Here's how the part is built. I have some questions about the finished solid (model axes, mm). Give positions to 0.01 mm unless a question says otherwise; leave off trailing zeros. Use CSV: the item, a comma, the result in double quotes. Start each with the question number.
(1) For pin 1 Ø2.5 at (x, z) = (50.42, -2.93) entering from -Y, with a flat end and sliding along its axis, tell me the tip position at first contact or that it passes through.
(2) Suppose I cut it at A-A on y = -0.5. Give the number of separate pieces and of enclosed holes in the cut face, plus the area to 3 significant figures.
(3) I need wall thicknesses on L1, parallel to X at y = -0.25, z = 15.5; L2, parallel to X at y = -1.35, z = -19.5; L3, parallel to X at y = -0.1, z = 6.5. Which ranges of each line are inside material? Lowest first, please. Write a range as [from, to].
from build123d import *

# Parameters (mm, degrees)
F0_R     = 1.857944
F0_R_2   = 1.417802
F0_R_3   = 1.435008
F0_R_4   = 1.79954
F0_R_5   = 1.437898
F0_R_6   = 1.231078
F0_R_7   = 1.385876
F0_R_8   = 1.711076
F0_R_9   = 1.741872
F0_R_10  = 1.225641
F0_R_11  = 1.503057
F0_R_12  = 1.860203
F0_R_13  = 1.749094
F0_R_14  = 1.743489
F0_R_15  = 1.494291
F0_R_16  = 1.596373
F0_R_17  = 1.637338
F1_DEPTH = 1.5875


with BuildPart() as f1:
    # F0 (on Front) → F1 (new body)
    with BuildSketch(Plane.XZ):
        with BuildLine():
            ThreePointArc((-53.66773, -11.336307), (-55.326937, -14.051365), (-57.893666, -15.931901))
            ThreePointArc((-57.893666, -15.931901), (-67.036765, -18.069861), (-74.114526, -24.240148))
            ThreePointArc((-74.114526, -24.240148), (-74.286866, -26.266206), (-73.075997, -27.899734))
            ThreePointArc((-73.075997, -27.899734), (-71.073113, -28.503398), (-69.070229, -27.899734))
            ThreePointArc((-69.070229, -27.899734), (-64.027702, -25.399624), (-58.438471, -24.73772))
            Line((-58.438471, -24.73772), (45.18429, -24.73772))
            ThreePointArc((45.18429, -24.73772), (58.781301, -21.232835), (68.98967, -11.591667))
            ThreePointArc((68.98967, -11.591667), (69.918229, -7.349726), (68.045994, -3.431687))
            ThreePointArc((68.045994, -3.431687), (64.632127, -2.335808), (61.21826, -3.431687))
            ThreePointArc((61.21826, -3.431687), (59.569704, -4.921663), (57.887653, -6.373721))
            ThreePointArc((57.887653, -6.373721), (56.415132, -3.677779), (54.260449, -1.488313))
            ThreePointArc((54.260449, -1.488313), (57.420268, 2.603666), (56.419311, 7.675828))
            ThreePointArc((56.419311, 7.675828), (53.426168, 9.07563), (50.251135, 8.16047))
            ThreePointArc((50.251135, 8.16047), (47.252127, 5.362267), (45.046306, 1.904182))
            ThreePointArc((45.046306, 1.904182), (37.452408, 4.595945), (29.940231, 1.68389))
            ThreePointArc((29.940231, 1.68389), (33.446145, 11.664014), (34.19633, 22.21539))
            ThreePointArc((34.19633, 22.21539), (32.218057, 24.773224), (29.015006, 24.329893))
            ThreePointArc((29.015006, 24.329893), (21.362188, 15.304458), (17.686093, 4.056772))
            ThreePointArc((17.686093, 4.056772), (15.865209, 4.289438), (14.044325, 4.056772))
            ThreePointArc((14.044325, 4.056772), (17.781783, 12.218199), (19.015627, 21.109493))
            ThreePointArc((19.015627, 21.109493), (16.476441, 24.638923), (12.194537, 23.884173))
            ThreePointArc((12.194537, 23.884173), (4.49603, 13.798937), (1.327041, 1.513316))
            ThreePointArc((1.327041, 1.513316), (-6.168675, 4.699529), (-13.66439, 1.513316))
            ThreePointArc((-13.66439, 1.513316), (-13.969566, 2.707403), (-14.243286, 3.909091))
            ThreePointArc((-14.243286, 3.909091), (-11.554331, 8.675915), (-14.82218, 13.066161))
            ThreePointArc((-14.82218, 13.066161), (-16.506238, 13.414686), (-18.190296, 13.066161))
            ThreePointArc((-18.190296, 13.066161), (-19.245169, 20.174848), (-24.033534, 25.533742))
            ThreePointArc((-24.033534, 25.533742), (-36.905205, 28.966058), (-49.776876, 25.533742))
            ThreePointArc((-49.776876, 25.533742), (-54.871128, 21.753364), (-58.402507, 16.483446))
            ThreePointArc((-58.402507, 16.483446), (-59.389188, 10.479151), (-57.068484, 4.854257))
            ThreePointArc((-57.068484, 4.854257), (-53.21663, 2.453173), (-48.687348, 2.157214))
            Line((-48.687348, 2.157214), (-53.66773, -11.336307))
        make_face()
        with Locations((-52.743013, -19.876236)):
            Circle(F0_R, mode=Mode.SUBTRACT)
        with Locations((-9.737349, -20.453916)):
            Circle(F0_R_2, mode=Mode.SUBTRACT)
        with BuildLine():
            Line((-27.557038, -14.726465), (-45.42472, -14.726465))
            ThreePointArc((-45.42472, -14.726465), (-42.378449, -9.519133), (-40.763168, -3.706479))
            ThreePointArc((-40.763168, -3.706479), (-33.288354, -4.538409), (-26.47082, -1.362535))
            ThreePointArc((-26.47082, -1.362535), (-25.533702, -2.36198), (-25.270261, -3.706479))
            ThreePointArc((-25.270261, -3.706479), (-27.322012, -7.146587), (-28.071562, -11.08133))
            ThreePointArc((-28.071562, -11.08133), (-28.011459, -12.931727), (-27.557038, -14.726465))
        make_face(mode=Mode.SUBTRACT)
        with Locations((-14.017423, -9.698912)):
            Circle(F0_R_3, mode=Mode.SUBTRACT)
        with BuildLine():
            ThreePointArc((-7.707629, -9.877752), (-9.432556, -8.514767), (-9.070634, -6.346331))
            ThreePointArc((-9.070634, -6.346331), (-6.806754, -8.318288), (-3.804479, -8.328883))
            ThreePointArc((-3.804479, -8.328883), (-5.599664, -9.49742), (-7.707629, -9.877752))
        make_face(mode=Mode.SUBTRACT)
        with Locations((-21.248184, -5.446013)):
            Circle(F0_R_4, mode=Mode.SUBTRACT)
        with Locations((-3.355453, -2.809598)):
            Circle(F0_R_5, mode=Mode.SUBTRACT)
        with Locations((48.567833, -20.610317)):
            Circle(F0_R_6, mode=Mode.SUBTRACT)
        with Locations((30.204914, -10.292606)):
            Circle(F0_R_7, mode=Mode.SUBTRACT)
        with Locations((3.54731, -6.039364)):
            Circle(F0_R_8, mode=Mode.SUBTRACT)
        with Locations((20.543733, -5.29803)):
            Circle(F0_R_9, mode=Mode.SUBTRACT)
        with Locations((65.664125, -7.364484)):
            Circle(F0_R_10, mode=Mode.SUBTRACT)
        with Locations((50.422841, -2.925415)):
            Circle(F0_R_11, mode=Mode.SUBTRACT)
        with Locations((-54.153713, 12.35175)):
            Circle(F0_R_12, mode=Mode.SUBTRACT)
        with Locations((-40.40785, 12.398653)):
            Circle(F0_R_13, mode=Mode.SUBTRACT)
        with BuildLine():
            ThreePointArc((-32.52355, 20.67507), (-29.489381, 18.275898), (-28.37258, 14.572526))
            ThreePointArc((-28.37258, 14.572526), (-29.043298, 9.932824), (-31.584578, 5.993461))
            ThreePointArc((-31.584578, 5.993461), (-34.573317, 4.144153), (-37.97367, 3.255278))
            Line((-37.97367, 3.255278), (-32.812039, 18.142183))
            ThreePointArc((-32.812039, 18.142183), (-32.514289, 19.391143), (-32.52355, 20.67507))
        make_face(mode=Mode.SUBTRACT)
        with Locations((-23.560752, 12.398653)):
            Circle(F0_R_14, mode=Mode.SUBTRACT)
        with BuildLine():
            ThreePointArc((-17.768233, 8.914482), (-16.558831, 9.198976), (-15.701279, 8.299981))
            ThreePointArc((-15.701279, 8.299981), (-16.9498, 7.883902), (-17.768233, 8.914482))
        make_face(mode=Mode.SUBTRACT)
        with BuildLine():
            ThreePointArc((-49.487693, 12.402402), (-47.245252, 17.284471), (-42.941975, 20.500827))
            ThreePointArc((-42.941975, 20.500827), (-45.655704, 14.868968), (-47.417419, 8.870758))
            ThreePointArc((-47.417419, 8.870758), (-48.41807, 9.229162), (-49.152797, 9.997231))
            ThreePointArc((-49.152797, 9.997231), (-49.493656, 11.175671), (-49.487693, 12.402402))
        make_face(mode=Mode.SUBTRACT)
        with Locations((39.767036, 0.559673)):
            Circle(F0_R_15, mode=Mode.SUBTRACT)
        with Locations((13.554551, 18.52873)):
            Circle(F0_R_16, mode=Mode.SUBTRACT)
        with Locations((29.518481, 18.52873)):
            Circle(F0_R_17, mode=Mode.SUBTRACT)
    extrude(amount=F1_DEPTH)


solid = f1.part
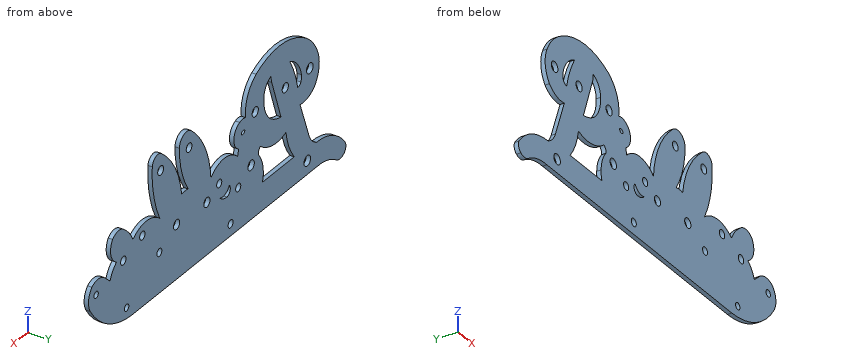
Geometry says:
1,pin 1,"through"
2,separate pieces,"1"
2,enclosed holes,"22"
2,area,"4,520 mm²"
3,L1,"[-58.81, -48.42], [-45.41, -33.73], [-28.43, -18.08], [5.39, 18.55], [21.47, 34.05]"
3,L2,"[-69.4, -54.56], [-50.92, -10.79], [-8.69, 48.04], [49.1, 61.53]"
3,L3,"[-58.15, -36.85], [-31.11, -11.9], [1.99, 15.47], [18.09, 32.01], [48.29, 57.08]"
